Geometry check sheet. Reference: the model listing, model coordinates, mm. A direction names the side the tool comes from. Round coordinates to 2 decimals unless told otherwise and drop trailing zeros. Order: outer loops, then holes, each group sorted by start corner. A loop starts at its lowest first (then second) coordinate and runs counter-clockwise, first axis right, second up. Notation, with made-up numbers: (-21.75, 79.25) - (-3.75, 79.25) arc R15 cw to (-3.75, 94.25) - close; hole circle Ø8 at (-29.5, 80). An arc over 180 degrees is marked (long way). Use a Markdown table: item, result. Add a question column.
(1) Section check A-A on z = 964. Record the boundary of the cut face in (x, y).
(2) Section check B-B on x = -161. Record the boundary of the cut face in (y, z), then the cut area to 3 significant figures.
(3) Access from +Z, -Z, +X, -X, +Y, -Y to the whole of each face (thin tool, end or side, straight path). Record for faces 4 (the face through (-573.939, 0.089, 884.738)), 5 (the face through (-364, -6.35, 975)).
(4) Section check D-D on x = -631.5. Record the boundary of the cut face in (y, z), then the cut area to 3 significant figures.
(5) Section check C-C on y = -0.25. Give the number of separate pieces and of enclosed holes in the cut face, then the cut area to 3 significant figures.
(6) Gauge pin test, flat ends, axial feed: P1, Ø5, axis at x = -571.75, z = 875.38, coming from the +Y side; P2, Ø4, axis at x = -402, y = 0.5, coming from the -Z side. Record the tip position at first contact, or that the pin passes through.
(7) Mould release check, pull along Z, two halves, no side actions. Record for faces 1 (the face through (-216.99, 0.09, 990.74)), 2 (the face through (-364, 6.35, 975)), 3 (the face through (-307, 0, 1014.879)): released by +Z, released by -Z, zero draft, split by the parting line, or undercut.
(8) Thickness scan on line 1 along Z through (x, y) = (-517.5, -5); line 2 along Z through (x, y) = (-265, 3.25); line 3 along Z through (x, y) = (-590, 1). Record the ranges inside material, lowest first. Write a range as [from, to].
```python
from build123d import *
from build123d.topology import SkipClean

# Parameters (mm, degrees)
SKETCH1_R           = 4.064
SKETCH1_R_2         = 3.2639
BOSS_EXTRUDE1_DEPTH = 6.35
CUT_EXTRUDE1_DEPTH  = 1227.767455485
FILLET1_R           = 5.08
FILLET2_R           = 1.27
FILLET3_R           = 2.54


with BuildPart() as part:
    # Sketch1 → Boss-Extrude1 (new, symmetric)
    with BuildSketch(Plane(origin=(0, 0, 0), x_dir=(1, 0, 0), z_dir=(0, 1, 0))):
        with BuildLine():
            Line((-580.023560274, -1020.213175904), (-32.743203186, -1020.213175904))
            ThreePointArc((-32.743203186, -1020.213175904), (-22.406526942, -1011.065872486), (-30.22862042, -999.693322674))
            Line((-30.22862042, -999.693322674), (-477.113436037, -888.497480987))
            ThreePointArc((-477.113436037, -888.497480987), (-477.140285594, -888.490838013), (-477.1671527, -888.484266374))
            Line((-477.1671527, -888.484266374), (-569.477932839, -866.035116584))
            ThreePointArc((-569.477932839, -866.035116584), (-569.495309073, -866.030907949), (-569.512693103, -866.026731636))
            Line((-569.512693103, -866.026731636), (-669.296750672, -842.152874275))
            ThreePointArc((-669.296750672, -842.152874275), (-679.306252785, -845.844627483), (-679.744367756, -856.504234867))
            Line((-679.744367756, -856.504234867), (-580.023560274, -1020.213175904))
        make_face()
        with Locations(Location((-32.743203186, -1009.799175904, 0), (0, 0, 270))):
            Circle(SKETCH1_R, mode=Mode.SUBTRACT)
        with Locations(Location((-479.628018803, -898.603334218, 0), (0, 0, 270))):
            Circle(SKETCH1_R, mode=Mode.SUBTRACT)
        with Locations(Location((-571.749732399, -875.37674385, 0), (0, 0, 270))):
            Circle(SKETCH1_R_2, mode=Mode.SUBTRACT)
        with Locations(Location((-671.533789968, -851.502886488, 0), (0, 0, 270))):
            Circle(SKETCH1_R_2, mode=Mode.SUBTRACT)
    extrude(amount=BOSS_EXTRUDE1_DEPTH, both=True)

    # Sketch2 → Cut-Extrude1 (cut, through all)
    with SkipClean():  # the faces are left unmerged after this step: merging them gives an invalid solid
        with BuildSketch(Plane(origin=(0, 6.35, 0), x_dir=(1, 0, 0), z_dir=(0, 1, 0))):
            with BuildLine():
                Line((-679.744367756, -856.504234867), (-580.023560274, -1020.213175904))
                Line((-580.023560274, -1020.213175904), (-32.743203186, -1020.213175904))
                ThreePointArc((-32.743203186, -1020.213175904), (-38.013320642, -1018.781227897), (-41.834132511, -1014.879175904))
                Line((-41.834132511, -1014.879175904), (-577.963867352, -1014.879175904))
                Line((-577.963867352, -1014.879175904), (-671.626154715, -861.116342785))
                ThreePointArc((-671.626154715, -861.116342785), (-676.282747595, -859.861981814), (-679.744367756, -856.504234867))
            make_face()
            with BuildLine():
                Line((-569.512693103, -866.026731636), (-669.296750672, -842.152874275))
                ThreePointArc((-669.296750672, -842.152874275), (-665.037914564, -844.415526194), (-662.413625342, -848.461559408))
                Line((-662.413625342, -848.461559408), (-578.505786805, -868.536948379))
                ThreePointArc((-578.505786805, -868.536948379), (-574.334431882, -866.116808548), (-569.512693103, -866.026731636))
            make_face()
            with BuildLine():
                Line((-469.57946129, -895.868761508), (-40.33850922, -1002.674379609))
                ThreePointArc((-40.33850922, -1002.674379609), (-35.688557552, -999.810367984), (-30.22862042, -999.693322674))
                Line((-30.22862042, -999.693322674), (-477.113436037, -888.497480987))
                ThreePointArc((-477.113436037, -888.497480987), (-472.345020276, -891.159589968), (-469.57946129, -895.868761508))
            make_face()
            with BuildLine():
                Line((-477.1671527, -888.484266374), (-569.477932839, -866.035116584))
                ThreePointArc((-569.477932839, -866.035116584), (-565.197857445, -868.341119656), (-562.593315725, -872.446367271))
                Line((-562.593315725, -872.446367271), (-487.201130908, -891.45495195))
                ThreePointArc((-487.201130908, -891.45495195), (-482.584369255, -888.617775245), (-477.1671527, -888.484266374))
            make_face()
            with BuildLine():
                ThreePointArc((-565.077216711, -882.298059303), (-574.043489966, -884.713003777), (-580.869897025, -878.41807093))
                Line((-580.869897025, -878.41807093), (-660.846200897, -859.283322179))
                Line((-660.846200897, -859.283322179), (-574.408981883, -1001.184956836))
                Line((-574.408981883, -1001.184956836), (-489.404527792, -902.190989161))
                ThreePointArc((-489.404527792, -902.190989161), (-489.554632834, -901.751941826), (-489.685031894, -901.306643982))
                Line((-489.685031894, -901.306643982), (-565.077216711, -882.298059303))
            make_face()
            Polygon((-196.508330191, -974.285316963), (-450.342933685, -911.125076565), (-302.454173976, -1004.719175904), align=None)
            with BuildLine():
                Line((-321.452940497, -1004.719175904), (-474.662853281, -907.757487774))
                ThreePointArc((-474.662853281, -907.757487774), (-478.086983606, -908.902684028), (-481.696350414, -908.809871355))
                Line((-481.696350414, -908.809871355), (-564.05205619, -1004.719175904))
                Line((-564.05205619, -1004.719175904), (-321.452940497, -1004.719175904))
            make_face()
            Polygon((-74.197736242, -1004.719175904), (-176.789592181, -979.191819922), (-265.654999436, -1004.719175904), align=None)
        extrude(amount=-CUT_EXTRUDE1_DEPTH, mode=Mode.SUBTRACT)

    # Fillet1
    fillet1_edges = [part.edges().sort_by_distance(p)[0] for p in [
        (-662.413625342, 0, 848.461559408),
        (-578.505786805, 0, 868.536948379),
        (-671.626154715, 0, 861.116342785),
        (-41.834132511, 0, 1014.879175904),
        (-302.454173976, 0, 1004.719175904),
        (-176.789592181, 0, 979.191819922),
        (-580.869897025, 0, 878.41807093),
        (-565.077216711, 0, 882.298059303),
        (-574.408981883, 0, 1001.184956836),
        (-469.57946129, 0, 895.868761508),
        (-40.33850922, 0, 1002.674379609),
        (-481.696350414, 0, 908.809871355),
        (-474.662853281, 0, 907.757487774),
        (-564.05205619, 0, 1004.719175904),
        (-562.593315725, 0, 872.446367271),
        (-487.201130908, 0, 891.45495195),
    ]]
    fillet(fillet1_edges, radius=FILLET1_R)

    # Fillet2
    fillet2_edges = [part.edges().sort_by_distance(p)[0] for p in [
        (-577.963867352, 0, 1014.879175904),
        (-450.342933685, 0, 911.125076565),
        (-196.508330191, 0, 974.285316963),
        (-74.197736242, 0, 1004.719175904),
        (-265.654999436, 0, 1004.719175904),
        (-660.846200897, 0, 859.283322179),
        (-321.452940497, 0, 1004.719175904),
    ]]
    fillet(fillet2_edges, radius=FILLET2_R)

    # Fillet3
    # the kernel refuses this fillet: 2.54 mm, written as the material it adds along each edge
    with BuildSketch(Plane(origin=(-489.685031894, 6.35, 901.306643982), x_dir=(-0.9696547275451901, 0, -0.24447844352675166), z_dir=(0, -1, 0))) as fillet3_piece_1:
        with BuildLine():
            CenterArc((3.223121953, -2.54), FILLET3_R, 90, 116.501118017)
            Line((0.95001079, -3.673386801), (0.722699673, -3.786725481))
            ThreePointArc((0.722699673, -3.786725481), (-0.715506578, -0.902270957), (-0.221729984, 0.123902439))
            Line((-0.221729984, 0.123902439), (0, 0.254))
            Line((0, 0.254), (3.223121953, 0.254))
            Line((3.223121953, 0.254), (3.223121953, 0))
        make_face()
    extrude(amount=12.7)
    with BuildSketch(Plane(origin=(-489.404527792, 6.35, 902.190989161), x_dir=(-0.6514647829655796, 0, 0.7586788757805311), z_dir=(0, -1, 0))) as fillet3_piece_2:
        with BuildLine():
            CenterArc((3.223121953, 2.54), FILLET3_R, 153.498881983, 116.501118017)
            Line((0.95001079, 3.673386801), (0.722699673, 3.786725481))
            ThreePointArc((0.722699673, 3.786725481), (-0.715506578, 0.902270957), (-0.221729984, -0.123902439))
            Line((-0.221729984, -0.123902439), (0, -0.254))
            Line((0, -0.254), (3.223121953, -0.254))
            Line((3.223121953, -0.254), (3.223121953, 0))
        make_face()
    extrude(amount=12.7)


solid = part.part
```
Check sheet entries:
| question | item | result |
|---|---|---|
| 1 | outline | (-608.96, -6.35) - (-597.06, -6.35) - (-597.06, 6.35) - (-608.96, 6.35) - close; (-542.48, -6.35) - (-529.09, -6.35) - (-529.09, 6.35) - (-542.48, 6.35) - close; (-385.79, -6.35) - (-366.79, -6.35) - (-366.79, 6.35) - (-385.79, 6.35) - close; (-237.84, -6.35) - (-195.77, -6.35) - (-195.77, 6.35) - (-237.84, 6.35) - close |
| 2 | outline | (-6.35, 972.65) - (6.35, 972.65) - (6.35, 983.12) - (-6.35, 983.12) - close; (-6.35, 1004.72) - (6.35, 1004.72) - (6.35, 1014.88) - (-6.35, 1014.88) - close |
| 2 | area | 262 mm2 |
| 3 | face 4 | +Y, -Y |
| 3 | face 5 | +Z, -Z, +X, -X, -Y |
| 4 | outline | (-6.35, 855.86) - (6.35, 855.86) - (6.35, 866.3) - (-6.35, 866.3) - close; (-6.35, 907.46) - (6.35, 907.46) - (6.35, 926.99) - (-6.35, 926.99) - close |
| 4 | area | 381 mm2 |
| 5 | separate pieces | 1 |
| 5 | enclosed holes | 8 |
| 5 | area | 18,500 mm2 |
| 6 | P1 | passes through |
| 6 | P2 | stops at z = 912.19 |
| 7 | face 1 | undercut |
| 7 | face 2 | zero draft |
| 7 | face 3 | released by +Z |
| 8 | line 1 | z = [883.82, 894.29], [934.91, 950.51], [1004.72, 1014.88] |
| 8 | line 2 | z = [946.77, 957.24], [993.96, 1014.88] |
| 8 | line 3 | z = [865.79, 876.23], [975.59, 995.12] |
